```python
from build123d import *

# Parameters (mm, degrees)
EXTRUDE_1_DEPTH     = 332
SKETCH_2_R          = 3.25
CUT_EXTRUDE_1_DEPTH = 5
SKETCH_3_R          = 5
CUT_EXTRUDE_2_DEPTH = 5
SKETCH_4_W          = 26.179083289
SKETCH_4_H          = 3.25731829
CUT_EXTRUDE_3_DEPTH = 10
SKETCH_5_R          = 1.75
CUT_EXTRUDE_4_DEPTH = 2.5
CHAMFER_1_SIZE      = 1.5
SKETCH_6_R          = 1.7
SKETCH_6_R_2        = 1.2
SKETCH_6_R_3        = 4
CUT_EXTRUDE_5_DEPTH = 10
SKETCH_7_R          = 2.1
CUT_EXTRUDE_6_DEPTH = 10


with BuildPart() as part:
    # Эскиз1 → Вытянуть1 (new body)
    with BuildSketch(Plane.XY):
        with BuildLine():
            Line((-1, -68), (-1, 104))
            ThreePointArc((-1, 104), (0.171572875, 106.828427125), (3, 108))
            Line((3, 108), (24, 108))
            Line((24, 108), (24, 106))
            Line((24, 106), (3, 106))
            ThreePointArc((3, 106), (1.585786438, 105.414213562), (1, 104))
            Line((1, 104), (1, -68))
            ThreePointArc((1, -68), (-0.171572875, -70.828427125), (-3, -72))
            Line((-3, -72), (-44, -72))
            Line((-44, -72), (-44, -70))
            Line((-44, -70), (-3, -70))
            ThreePointArc((-3, -70), (-1.585786438, -69.414213562), (-1, -68))
        make_face()
    extrude(amount=EXTRUDE_1_DEPTH)

    # Эскиз2 → Вырез-Вытянуть1 (cut)
    with BuildSketch(Plane.ZY.offset(1)):
        with Locations((31, -38)):
            Circle(SKETCH_2_R)
        with Locations((121, -38)):
            Circle(SKETCH_2_R)
        with Locations((211, -38)):
            Circle(SKETCH_2_R)
        with Locations((301, -38)):
            Circle(SKETCH_2_R)
    extrude(amount=-CUT_EXTRUDE_1_DEPTH, mode=Mode.SUBTRACT)

    # Эскиз3 → Вырез-Вытянуть2 (cut)
    with BuildSketch(Plane(origin=(0, -70, 0), x_dir=(1, 0, 0), z_dir=(0, 1, 0))):
        with Locations(Location((-24, -18.5, 0), (0, 0, 270))):
            Circle(SKETCH_3_R)
        with Locations(Location((-24, -313.5, 0), (0, 0, 270))):
            Circle(SKETCH_3_R)
    extrude(amount=-CUT_EXTRUDE_2_DEPTH, mode=Mode.SUBTRACT)

    # Эскиз4 → Вырез-Вытянуть3 (cut)
    with BuildSketch(Plane(origin=(0, 108, 0), x_dir=(1, 0, 0), z_dir=(0, 1, 0))):
        with Locations((16.089541645, 0.628659145)):
            Rectangle(SKETCH_4_W, SKETCH_4_H)
        with Locations((16.089541645, -332.628659145)):
            Rectangle(SKETCH_4_W, SKETCH_4_H)
    extrude(amount=-CUT_EXTRUDE_3_DEPTH, mode=Mode.SUBTRACT)

    # Эскиз5 → Вырез-Вытянуть4 (cut)
    with BuildSketch(Plane.ZY.offset(1)):
        with Locations(Location((5.7, 95, 0), (0, 0, 270))):
            Circle(SKETCH_5_R)
        with Locations(Location((326.3, 95, 0), (0, 0, 270))):
            Circle(SKETCH_5_R)
    extrude(amount=-CUT_EXTRUDE_4_DEPTH, mode=Mode.SUBTRACT)

    # Фаска1
    chamfer_1_edges = [part.edges().sort_by_distance(p)[0] for p in [
        (-1, 96.75, 326.3),
        (-1, 96.75, 5.7),
    ]]
    chamfer(chamfer_1_edges, length=CHAMFER_1_SIZE)

    # Эскиз6 → Вырез-Вытянуть5 (cut)
    with BuildSketch(Plane.ZY.offset(1)):
        with Locations(Location((257, 55.5, 0), (0, 0, 270))):
            Circle(SKETCH_6_R)
        with Locations(Location((304, 55.5, 0), (0, 0, 270))):
            Circle(SKETCH_6_R)
        with Locations(Location((258.5, 10, 0), (0, 0, 270))):
            Circle(SKETCH_6_R_2)
        with Locations(Location((302.5, 10, 0), (0, 0, 270))):
            Circle(SKETCH_6_R_2)
        with Locations(Location((271.5, 5, 0), (0, 0, 270))):
            Circle(SKETCH_6_R_3)
        with Locations(Location((289.5, 5, 0), (0, 0, 270))):
            Circle(SKETCH_6_R_3)
        with BuildLine():
            Line((260.14870942, 51.635803619), (260.875982147, 59.635803619))
            ThreePointArc((260.875982147, 59.635803619), (261.358314525, 60.607633836), (262.369821957, 61))
            Line((262.369821957, 61), (298.630178043, 61))
            ThreePointArc((298.630178043, 61), (299.641685475, 60.607633836), (300.124017853, 59.635803619))
            Line((300.124017853, 59.635803619), (300.85129058, 51.635803619))
            ThreePointArc((300.85129058, 51.635803619), (300.465084606, 50.488492568), (299.35745077, 50))
            Line((299.35745077, 50), (261.64254923, 50))
            ThreePointArc((261.64254923, 50), (260.534915394, 50.488492568), (260.14870942, 51.635803619))
        make_face()
    extrude(amount=-CUT_EXTRUDE_5_DEPTH, mode=Mode.SUBTRACT)

    # Эскиз7 → Вырез-Вытянуть6 (cut)
    with BuildSketch(Plane(origin=(0, 108, 0), x_dir=(1, 0, 0), z_dir=(0, 1, 0))):
        with Locations(Location((13.353335267, -166, 0), (0, 0, 270))):
            Circle(SKETCH_7_R)
        with Locations(Location((13, -15, 0), (0, 0, 270))):
            Circle(SKETCH_7_R)
        with Locations(Location((13, -317, 0), (0, 0, 270))):
            Circle(SKETCH_7_R)
    extrude(amount=-CUT_EXTRUDE_6_DEPTH, mode=Mode.SUBTRACT)


solid = part.part
```
Build history of the part. All positions in model axes, mm. A direction names the side the tool comes from. Coordinates: 2 decimals unless noted, no trailing zeros. Order: outer loops, then holes, each group sorted by start corner. A loop starts at its lowest first (then second) coordinate and runs counter-clockwise, first axis right, second up. Notation, with made-up numbers: (40.5, 35.5) -> (67.5, 35.5) arc R7 cw to (67.5, 41.5) -> close; hole circle Ø9 at (-36.75, 78). An arc over 180 degrees is marked (long way). Answer in a Markdown table with one row per item. Add a question column.
Q1. Band-saw the part on B-B, the plane z = 289.5. List the corners of the cut face in (x, y), then the cut area to 3 significant figures.
Q2. Band-saw the part on A-A, the plane y = 5. List the corners of the cut face in (x, z), then the cut area to 3 significant figures.
Q3. Mould opens along Y. For faces 4 (the face through (-24, -70, 164)), 5 (the face through (0, 18, 332)), 6 (the face through (-23, -72, 164)), 7 (the face through (-0.014, 3.154, 285.951)) say: +Y half, -Y half, draft (parallel to the pull), parting line (faces both ways), or undercut.
Q4. Band-saw the part on D-D, the plane z = 31. List the corners of the cut face in (x, y).
Q5. Drop flat-ended pins along their axis: pin 1 (12 mm diameter, centred on x = -15, z = 214, fed in from +Y); pin 2 (3 mm diameter, centred on x = -0.5, z = 215, fed in from +Y); pin 3 (1 mm diameter, centred on x = 0, z = 275.5, fed in from -Y). Give the stop position or say it passes through.
Q6. Which spindle directions (+Z, -Z, +X, -X, +Y, -Y) get a long thin tool onto all of the face, cutting with end or side? Do faces 1 (the face through (1, 19, 164)), 2 (the face through (-1, 17, 164)), 3 (the face through (-28.88, -70.99, 17.42)). Say none if no direction does.
Q7. Band-saw the part on C-C, the plane y = -38. List the corners of the cut face in (x, z).
Q8. Wall check: line 1 along Z through (x, y) = (0.55, 5); line 2 along X through (y, z) = (17, 208); line 3 along Y through (x, z) = (-38.5, 95). Give the ranges that are in metal, low to high. Write a range as [from, to].
Answers follow:
| question | item | result |
|---|---|---|
| 1 | outline | (-44, -72) -> (-3, -72) arc R4 ccw to (1, -68) -> (1, 1) -> (-1, 1) -> (-1, -68) arc R2 cw to (-3, -70) -> (-44, -70) -> close; (-1, 9) -> (1, 9) -> (1, 50) -> (-1, 50) -> close; (-1, 61) -> (1, 61) -> (1, 104) arc R2 cw to (3, 106) -> (24, 106) -> (24, 108) -> (3, 108) arc R4 ccw to (-1, 104) -> close |
| 1 | area | 449 mm^2 |
| 2 | outline | (-1, 0) -> (1, 0) -> (1, 267.5) -> (-1, 267.5) -> close; (-1, 275.5) -> (1, 275.5) -> (1, 285.5) -> (-1, 285.5) -> close; (-1, 293.5) -> (1, 293.5) -> (1, 332) -> (-1, 332) -> close |
| 2 | area | 632 mm^2 |
| 3 | face 4 | +Y half |
| 3 | face 5 | draft |
| 3 | face 6 | -Y half |
| 3 | face 7 | undercut |
| 4 | outline | (-44, -72) -> (-3, -72) arc R4 ccw to (1, -68) -> (1, -41.25) -> (-1, -41.25) -> (-1, -68) arc R2 cw to (-3, -70) -> (-44, -70) -> close; (-1, -34.75) -> (1, -34.75) -> (1, 104) arc R2 cw to (3, 106) -> (24, 106) -> (24, 108) -> (3, 108) arc R4 ccw to (-1, 104) -> close |
| 5 | pin 1 | y = -70 |
| 5 | pin 2 | y = 107.46 |
| 5 | pin 3 | y = -71.12 |
| 6 | face 1 | +Z, -Z, +X, -Y |
| 6 | face 2 | +Z, -Z, -X, +Y |
| 6 | face 3 | +Y, -Y |
| 7 | outline | (-1, 0) -> (1, 0) -> (1, 27.75) -> (-1, 27.75) -> close; (-1, 34.25) -> (1, 34.25) -> (1, 117.75) -> (-1, 117.75) -> close; (-1, 124.25) -> (1, 124.25) -> (1, 207.75) -> (-1, 207.75) -> close; (-1, 214.25) -> (1, 214.25) -> (1, 297.75) -> (-1, 297.75) -> close; (-1, 304.25) -> (1, 304.25) -> (1, 332) -> (-1, 332) -> close |
| 8 | line 1 | [0, 267.5], [275.5, 285.5], [293.5, 332] |
| 8 | line 2 | [-1, 1] |
| 8 | line 3 | [-72, -70] |
